Part model, mm, in its own coordinate system. Face numbers are marked on the shaded views. A direction names the side the tool comes from. Coordinates: 2 decimals unless noted, no trailing zeros. Write each loop counter-clockwise with the first axis right and the second up, starting at its lowest first coordinate (ties: lowest second). Pieces come first, ordered by that corner, then holes. Notation, with made-up numbers: (82, 67.5) -> (87, 67.5) arc R16 cw to (87, 86.5) -> close; hole circle Ø4 at (80.5, 58). An arc over 180 degrees is marked (long way). One line per question, with ' | ' between items. Start each with the question number.
Item 1: Saw through at B-B (z = 74). List the corners of the cut face in (x, y), and give its area (3 significant figures).
Item 2: Two-plate mould, pull along Y, no slides. Class the marked faces 1, 2 and 3: pulls with the +Y half, pulls with the -Y half, needs draft (parallel to the pull), parting line crosses it, or undercut.
Item 3: Saw through at A-A (x = 63.5). List the corners of the cut face in (y, z).
Item 4: Probe probe 1 along Y at (x, z) = (63.5, 5.75); probe 2 along Z at (x, y) = (109, -40.5); probe 3 along X at (y, z) = (-11.5, 70). List the from-to ranges inside material, lowest first. Write a range as [from, to].
Item 5: Saw through at D-D (z = 33.5). List the corners of the cut face in (x, y).
Item 6: Saw through at C-C (y = -71). List the corners of the cut face in (x, z), and give its area (3 significant figures).
Item 7: Pin check, flat tips, straight feed: pin 1 (5 mm diameter, centred on y = -74, z = 76.5, fed in from +X); pin 2 (2 mm diameter, centred on x = 167.5, y = -27.5, fed in from +Z); pin 3 (12 mm diameter, centred on y = -56, z = 43, fed in from -X). Stop position of each tip, or through.
Item 8: 3-axis set-ups, long thin cutter, end or side, ignore diameter. For the marked faces 4 and 5: which of +Z, -Z, +X, -X, +Y, -Y reach the whole face in a straight line?
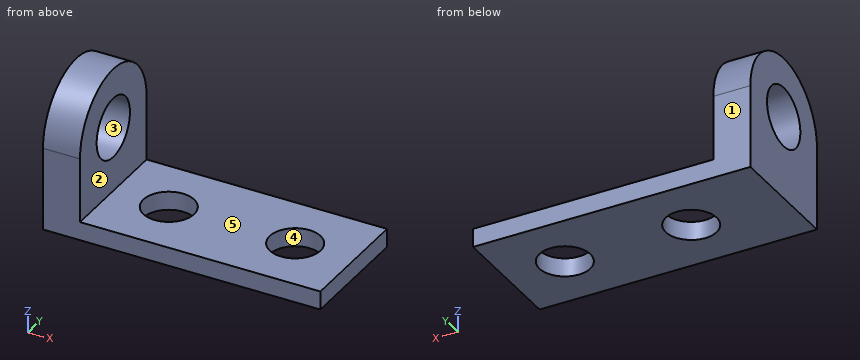
from build123d import *

# Parameters (mm, degrees)
F1_DEPTH = 82.55
F2_R     = 17.4625
F3_DEPTH = 25.4
F5_DEPTH = 25.4
F6_R     = 20.6375
F7_DEPTH = 25.4


with BuildPart() as f1:
    # F0 (on Front) → F1 (new body)
    with BuildSketch(Plane.XZ):
        Polygon((0, 107.95), (0, 0), (190.5, 0), (190.5, 12.7), (25.4, 12.7), (25.4, 107.95), align=None)
    extrude(amount=F1_DEPTH)

    # F2 (on face) → F3 (cut)
    with BuildSketch(Plane.XY.offset(12.7)):
        with Locations((63.5, -41.275)):
            Circle(F2_R)
        with Locations((150.305644, -41.275)):
            Circle(F2_R)
    extrude(amount=-F3_DEPTH, mode=Mode.SUBTRACT)

    # F4 (on face) → F5 (cut)
    with BuildSketch(Plane(origin=(0, 0, 0), x_dir=(0, -1, 0), z_dir=(-1, 0, 0))):
        with BuildLine():
            ThreePointArc((0, 57.15), (41.275, 98.425), (82.55, 57.15))
            Line((82.55, 57.15), (82.55, 107.95))
            Line((82.55, 107.95), (0, 107.95))
            Line((0, 107.95), (0, 57.15))
        make_face()
    extrude(amount=-F5_DEPTH, mode=Mode.SUBTRACT)

    # F6 (on face) → F7 (cut, through all)
    with BuildSketch(Plane(origin=(0, 0, 0), x_dir=(0, -1, 0), z_dir=(-1, 0, 0))):
        with Locations((41.275, 57.15)):
            Circle(F6_R)
    extrude(amount=-F7_DEPTH, mode=Mode.SUBTRACT)


solid = f1.part
From the geometry:
1) outline: (0, -78.95) -> (25.4, -78.95) -> (25.4, -53.19) -> (0, -53.19) -> close; (0, -29.36) -> (25.4, -29.36) -> (25.4, -3.6) -> (0, -3.6) -> close | area: 1,310 mm2
2) face 1: pulls with the +Y half | face 2: needs draft | face 3: undercut
3) outline: (-82.55, 0) -> (-58.74, 0) -> (-58.74, 12.7) -> (-82.55, 12.7) -> close; (-23.81, 0) -> (0, 0) -> (0, 12.7) -> (-23.81, 12.7) -> close
4) probe 1: [-82.55, -58.74], [-23.81, 0] | probe 2: [0, 12.7] | probe 3: [0, 25.4]
5) outline: (0, -82.55) -> (25.4, -82.55) -> (25.4, 0) -> (0, 0) -> close
6) outline: (0, 0) -> (190.5, 0) -> (190.5, 12.7) -> (25.4, 12.7) -> (25.4, 85.79) -> (0, 85.79) -> close | area: 4,280 mm2
7) pin 1: x = 25.4 | pin 2: z = 12.7 | pin 3: x = 0
8) face 4: +Z, -Z | face 5: +Z, +X, +Y, -Y
